Autodesk Inventor part; units mm, degrees
ref_plane "YZ Plane" through (0, 0, 0) normal (1, 0, 0) x (0, 1, 0)
ref_plane "XZ Plane" through (0, 0, 0) normal (0, 1, 0) x (-1, 0, 0)
ref_plane "XY Plane" through (0, 0, 0) normal (0, 0, 1) x (1, 0, 0)
sketch "Sketch1" plane through (0, 0, 0) normal (0, 0, 1) x (1, 0, 0)
  circle A0 centre (0, 0) radius 10
  dimension "d0" = 20
extrude "Extrusion1" add sketch "Sketch1" along normal blind 2.77
sketch "Sketch2" plane through (0, 0, 2.77) normal (0, 0, 1) x (1, 0, 0)
  circle A0 centre (0, 0) radius 2.5
  circle A1 centre (0, 0) radius 4.5
  dimension "d3" = 5
  dimension "d4" = 9
extrude "Extrusion2" add sketch "Sketch2" along normal blind 3
sketch "Sketch3" plane through (0, 0, 0) normal (0, 0, -1) x (-1, 0, 0)
  circle A0 centre (7.2, 0) radius 0.9
  circle A1 centre (0, 7.2) radius 0.9
  circle A2 centre (-7.2, 0) radius 0.9
  circle A3 centre (0, -7.2) radius 0.9
  point P0 (0, 0)
  dimension "d11" = 360
extrude "Extrusion3" cut sketch "Sketch3" against normal blind 3
sketch "Sketch4" plane through (0, 0, 0) normal (0, 0, -1) x (-1, 0, 0)
  circle A0 centre (0, 0) radius 2
  dimension "d18" = 4
extrude "Extrusion4" cut sketch "Sketch4" against normal blind 5
sketch "Sketch5" plane through (0, 0, 0) normal (0, 0, -1) x (-1, 0, 0)
  point P0 (0, 0)
equation "\"d16\" = d15"
properties part number "SERVOHORN"
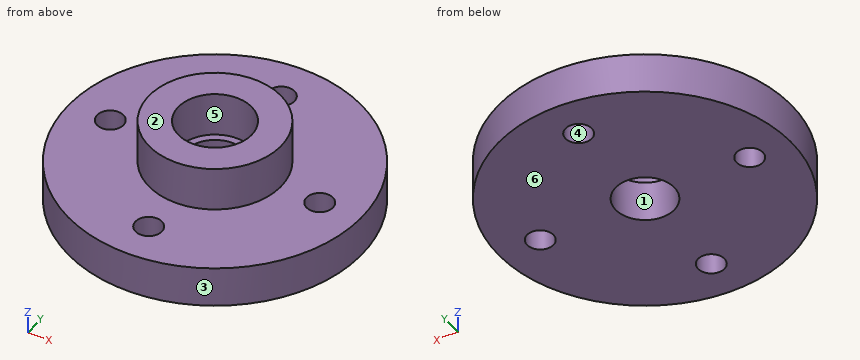
The model under review builds one solid part; all positions refer to its coordinate system, in mm. Face numbers are marked on the shaded views. A direction names the side the tool comes from. Coordinates: 2 decimals unless noted, no trailing zeros. Loops run counter-clockwise (first coordinate to the right, second up) from the corner with the lowest first, then second, coordinate; pieces in that order, holes last. Notation, with made-up numbers: (63, -34) -> (87, -34) arc R29 cw to (87, -9) -> close; hole circle Ø6 at (67.25, -2). An arc over 180 degrees is marked (long way). Use a Markdown table: item, result. Add a question column.
1. To check wall thickness, follow line 1 (Z direction, x = 8.5, y = 1.75); line 2 (Y direction, x = 1, z = 4); line 3 (Y direction, x = 7.25, z = 0.45). State the ranges of each line that lie inside material, in increasing order.
2. Draft analysis for pull direction Y (two halves, no side actions). For the marked faces 1, 2, 3 and 4, state which applies: pulls with the +Y half, pulls with the -Y half, needs draft (parallel to the pull), parting line crosses it, or undercut.
3. Clearance check with flat-ended pins moving along their axes: pin 1 Ø1.6 at (x, y) = (0, -7.2) entering from -Z; pin 2 Ø1 at (x, y) = (3.5, -6.5) entering from +Z; pin 3 Ø3 at (y, z) = (2.5, 2) entering from +X; pin 4 Ø2 at (x, z) = (-7.5, 3.5) entering from -Y. State where each tip first meets the part, or that it passes through.
4. Add section D-D on y = -7.2. Write out the cut boundary in (x, z).
5. Add section C-C on z = 1. Write out the cut boundary in (x, y).
6. Add section A-A on y = 0. Write out the cut boundary in (x, z).
7. Machinability: for the marked faces 5 and 6, which of the approach directions +Z, -Z, +X, -X, +Y, -Y give a long, thin tool a straight path to every point of the face, cutting with its end or side? Answer none if there is none.
Returned:
| question | item | result |
|---|---|---|
| 1 | line 1 | z = 0 to 2.77 |
| 1 | line 2 | y = -4.39 to -2.29, 2.29 to 4.39 |
| 1 | line 3 | y = -6.89 to -0.9, 0.9 to 6.89 |
| 2 | face 1 | undercut |
| 2 | face 2 | needs draft |
| 2 | face 3 | parting line crosses it |
| 2 | face 4 | undercut |
| 3 | pin 1 | passes through |
| 3 | pin 2 | stops at z = 2.77 |
| 3 | pin 3 | stops at x = 9.95 |
| 3 | pin 4 | stops at y = -7.32 |
| 4 | outline | (-6.94, 0) -> (-0.9, 0) -> (-0.9, 2.77) -> (-6.94, 2.77) -> close; (0.9, 0) -> (6.94, 0) -> (6.94, 2.77) -> (0.9, 2.77) -> close |
| 5 | outline | circle Ø20 at (0, 0); hole circle Ø1.8 at (-7.2, 0); hole circle Ø4 at (0, 0); hole circle Ø1.8 at (0, -7.2); hole circle Ø1.8 at (0, 7.2); hole circle Ø1.8 at (7.2, 0) |
| 6 | outline | (-10, 0) -> (-8.1, 0) -> (-8.1, 2.77) -> (-10, 2.77) -> close; (-6.3, 0) -> (-2, 0) -> (-2, 2.77) -> (-2.5, 2.77) -> (-2.5, 5.77) -> (-4.5, 5.77) -> (-4.5, 2.77) -> (-6.3, 2.77) -> close; (2, 0) -> (6.3, 0) -> (6.3, 2.77) -> (4.5, 2.77) -> (4.5, 5.77) -> (2.5, 5.77) -> (2.5, 2.77) -> (2, 2.77) -> close; (8.1, 0) -> (10, 0) -> (10, 2.77) -> (8.1, 2.77) -> close |
| 7 | face 5 | +Z |
| 7 | face 6 | -Z, +X, -X, +Y, -Y |
